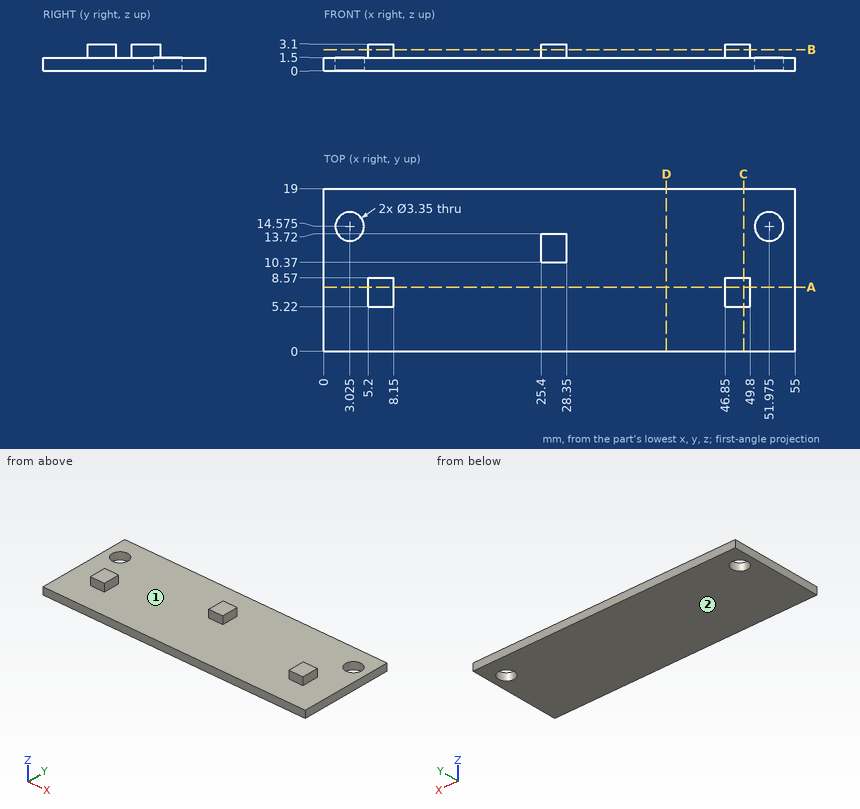
Study the drawing (mm; zero at the part's minimum x, y, z) and answer. Round coordinates to 2 decimals unless told otherwise and drop trailing zeros. Order: outer loops, then holes, each group sorted by start corner. A loop starts at its lowest first (then second) coordinate and runs counter-clockwise, first axis right, second up. Notation, with made-up numbers: (56, 36.25) - (105, 36.25) arc R22 ccw to (105, 75.25) - close; hole circle Ø2 at (59, 1.5). An arc over 180 degrees is marked (long way). Use one line per item in the form item = value. Start each with the question number.
(1) Flat-ended cylindrical pins translate along their axes: pin 1 Ø1.3 at (y, z) = (6.5, 2.5) entering from -X; pin 2 Ø0.8 at (y, z) = (12, 2.5) entering from -X; pin 3 Ø0.5 at (y, z) = (6, 2.5) entering from +X; pin 4 Ø3 at (x, y) = (51.975, 14.575) entering from +Z. Find the tip coordinate at first contact, or state that the pin passes through.
(2) The part is cut by section B-B (z = 2.45). Give the vertices of the cut face in (x, y), then the cut area to 3 significant figures.
(3) The part is cut by section A-A (y = 7.5). Give the vertices of the cut face in (x, z).
(4) Find the intervals of material crossed by line 1 along X through (y, z) = (14.5, 1.1); line 2 along X through (y, z) = (13.25, 1.3); line 3 along Z through (x, y) = (46, 13.5), in increasing order. Write a range as from..to.
(5) The part is cut by section D-D (x = 40). Give the vertices of the cut face in (y, z), then the cut area to 3 significant figures.
(6) The part is cut by section C-C (x = 49). Give the vertices of the cut face in (y, z).
(7) Determine the mould class of the marked faces 1 and 2 for opening direction X: +X half, -X half, draft (parallel to the pull), parting line (faces both ways), or undercut.
Checked values:
q1.pin_1 = 5.2
q1.pin_2 = 25.4
q1.pin_3 = 49.8
q1.pin_4 = through
q2.outline = (5.2, 5.22) - (8.15, 5.22) - (8.15, 8.57) - (5.2, 8.57) - close; (25.4, 10.37) - (28.35, 10.37) - (28.35, 13.72) - (25.4, 13.72) - close; (46.85, 5.22) - (49.8, 5.22) - (49.8, 8.57) - (46.85, 8.57) - close
q2.area = 29.6 mm^2
q3.outline = (0, 0) - (55, 0) - (55, 1.5) - (49.8, 1.5) - (49.8, 3.1) - (46.85, 3.1) - (46.85, 1.5) - (8.15, 1.5) - (8.15, 3.1) - (5.2, 3.1) - (5.2, 1.5) - (0, 1.5) - close
q4.line_1 = 0..1.35, 4.7..50.3, 53.65..55
q4.line_2 = 0..2, 4.05..50.95, 53..55
q4.line_3 = 0..1.5
q5.outline = (0, 0) - (19, 0) - (19, 1.5) - (0, 1.5) - close
q5.area = 28.5 mm^2
q6.outline = (0, 0) - (19, 0) - (19, 1.5) - (8.57, 1.5) - (8.57, 3.1) - (5.22, 3.1) - (5.22, 1.5) - (0, 1.5) - close
q7.face_1 = undercut
q7.face_2 = draft
